Verification items for the finished model (mm, model axes). Face numbers are marked on the shaded views. A direction names the side the tool comes from. Round coordinates to 2 decimals unless told otherwise and drop trailing zeros. Write each loop counter-clockwise with the first axis right and the second up, starting at its lowest first coordinate (ties: lowest second). Pieces come first, ordered by that corner, then holes.
from build123d import *

# Parameters (mm, degrees)
F0_R     = 4
F1_DEPTH = 50
F2_R     = 3.5
F3_DEPTH = 2.001
F4_W     = 15
F4_H     = 10
F5_DEPTH = 25
F6_R     = 4
F7_DEPTH = 50


with BuildPart() as f1:
    # F0 (on Front) → F1 (new body)
    with BuildSketch(Plane.XZ):
        with BuildLine():
            Line((26.190159, 30.504479), (0.662295, 30.504479))
            ThreePointArc((0.662295, 30.504479), (-6.259331, 39.981705), (-3.809841, 28.504479))
            Line((-3.809841, 28.504479), (26.190159, 28.504479))
            Line((26.190159, 28.504479), (26.190159, 30.504479))
        make_face()
        with Locations((-3.809841, 34.504479)):
            Circle(F0_R, mode=Mode.SUBTRACT)
    extrude(amount=F1_DEPTH)

    # F2 (on face) → F3 (cut, through all)
    with BuildSketch(Plane.XY.offset(30.504479)):
        with Locations((19.190159, -32)):
            Circle(F2_R)
        with Locations((9.190159, -44)):
            Circle(F2_R)
        with Locations((9.190159, -20)):
            Circle(F2_R)
        with Locations((19.190159, -8)):
            Circle(F2_R)
    extrude(amount=-F3_DEPTH, mode=Mode.SUBTRACT)

    # F4 (on face) → F5 (cut)
    with BuildSketch(Plane(origin=(0, 0, 28.504479), x_dir=(1, 0, 0), z_dir=(0, 0, -1))):
        with Locations((-4.309841, 35)):
            Rectangle(F4_W, F4_H)
        with Locations((-4.309841, 15)):
            Rectangle(F4_W, F4_H)
    extrude(amount=-F5_DEPTH, mode=Mode.SUBTRACT)

    # F6 (on face) → F7 (join)
    with BuildSketch(Plane(origin=(0, 0, 0), x_dir=(-1, 0, 0), z_dir=(0, 1, 0))):
        with Locations((3.809841, 34.504479)):
            Circle(F6_R)
    extrude(amount=-F7_DEPTH)


solid = f1.part
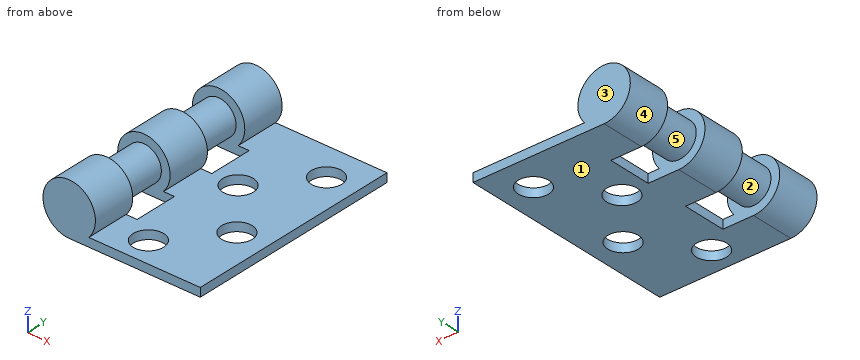
Q1. Sectioned sample at A-A (y = -8). Enter the section's corners in (x, z).
Recorded:
outline: (-3.81, 28.5) - (15.69, 28.5) - (15.69, 30.5) - (0.66, 30.5) arc R6 ccw (long way) to start; (22.69, 28.5) - (26.19, 28.5) - (26.19, 30.5) - (22.69, 30.5) - close
Q2. Material ranges on line 1 along Y through (x, z) = (-8, 35); line 2 along Z through (x, y) = (18, -43); line 3 along Y through (x, z) = (21.5, 29.25), recorded low to high.
Recorded:
line 1: y = -50 to -40, -30 to -20, -10 to 0
line 2: z = 28.5 to 30.5
line 3: y = -50 to -34.63, -29.37 to -10.63, -5.37 to 0
Q3. Sectioned sample at B-B (x = 17). Enter the section's corners in (y, z).
Recorded:
outline: (-50, 28.5) - (-34.73, 28.5) - (-34.73, 30.5) - (-50, 30.5) - close; (-29.27, 28.5) - (-10.73, 28.5) - (-10.73, 30.5) - (-29.27, 30.5) - close; (-5.27, 28.5) - (0, 28.5) - (0, 30.5) - (-5.27, 30.5) - close
Q4. Tool access check on the marked faces 4 and 5. Record the directions out of +Z, -Z, +X, -X, +Y, -Y that give a thin tool (end or side, any length) a straight path to the whole face; none if there is none.
Recorded:
face 4: +Y, -Y
face 5: none
Q5. Sectioned sample at D-D (z = 39.75). Enter the section's corners in (x, y), plus the area to 3 significant figures.
Recorded:
outline: (-6.72, -50) - (-0.9, -50) - (-0.9, -40) - (-6.72, -40) - close; (-6.72, -30) - (-0.9, -30) - (-0.9, -20) - (-6.72, -20) - close; (-6.72, -10) - (-0.9, -10) - (-0.9, 0) - (-6.72, 0) - close
area: 175 mm2
Q6. Release check for a two-part mould opening along Z. For the marked faces 1, 2 and 3 record: released by +Z, released by -Z, zero draft, split by the parting line, or undercut.
Recorded:
face 1: released by -Z
face 2: split by the parting line
face 3: zero draft
Q7. Sectioned sample at C-C (y = -18.5). Enter the section's corners in (x, z), plus the area to 3 significant figures.
Recorded:
outline: circle Ø8 at (-3.81, 34.5); (3.19, 28.5) - (6.03, 28.5) - (6.03, 30.5) - (3.19, 30.5) - close; (12.35, 28.5) - (26.19, 28.5) - (26.19, 30.5) - (12.35, 30.5) - close
area: 83.6 mm2
Q8. Depth check by flat-ended pin: P1, Ø1.5, axis at x = 14, y = -42, coming from the +Z side; P2, Ø6.5, axis at x = 19.19, y = -8, coming from the +Z side. Enter the tip coordinate at first touch or a pass-through.
Recorded:
P1: stops at z = 30.5
P2: passes through
